Input: part model. Units: mm. Frame: model coordinates. A direction names the side the tool comes from. Give positions to 0.01 mm unless a question says otherwise; leave off trailing zeros. Loops run counter-clockwise (first coordinate to the right, second up) from the corner with the lowest first, then second, coordinate; pieces in that order, holes last. Notation, with made-up numbers: (10, -38.75) - (37, -38.75) arc R30 ccw to (37, -5.75) - close; hole circle Ø9 at (19.25, 66). An arc over 180 degrees is marked (long way). One line per item, written item: value.
from build123d import *

# Parameters (mm, degrees)
SKETCH_2_W               = 28
SKETCH_2_H               = 4.5
CUT_EXTRUDE_1_DEPTH      = 10
EXTRUDE_1_DEPTH          = 15
HOLE_WIZARD_M3_1_D       = 2.5
HOLE_WIZARD_M3_1_DEPTH   = 4
HOLE_WIZARD_M3_1_TIP     = 0.751075774
CUT_EXTRUDE_START        = -20
CUT_EXTRUDE_2_DEPTH      = 20
HOLE_WIZARD_M4_1_D       = 3.3
HOLE_WIZARD_M4_1_DEPTH   = 10.1
HOLE_WIZARD_M4_1_TIP     = 0.991420021
CUT_EXTRUDE_3_DEPTH      = 64.617293246
CUT_EXTRUDE_3_DEPTH_BACK = 64.617293246
SKETCH_11_R              = 1.5


with BuildPart() as part:
    # 草图1 → 旋转1 (revolve)
    with BuildSketch(Plane.XY, mode=Mode.PRIVATE) as revolve_1_sk:
        Polygon((0, 0), (4.1, 0), (4.1, 6.7), (13.4, 6.7), (13.4, 8.7), (21, 8.7), (21, 10.2), (20, 10.2), (20, 11.2), (21, 11.2), (21, 12.2), (10, 12.2), (10, 13.2), (21, 13.2), (21, 20.4), (5, 20.4), (5, 21), (21, 21), (21, 34.7), (18.3, 38.7), (3.5, 38.7), (3.5, 43.7), (0, 43.7), align=None)
    revolve(revolve_1_sk.sketch.rotate(Axis((0, 43.7, 0), (0, -1, 0)), 90), axis=Axis((0, 43.7, 0), (0, -1, 0)))

    # 草图2 → 切除-拉伸1 (cut)
    with BuildSketch(Plane.XY.offset(21)):
        with Locations((0, 16.05)):
            Rectangle(SKETCH_2_W, SKETCH_2_H)
    extrude(amount=-CUT_EXTRUDE_1_DEPTH, mode=Mode.SUBTRACT)

    # 草图3 → 凸台-拉伸1 (add)
    with BuildSketch(Plane.XY.offset(11)):
        with BuildLine():
            Line((9.185056323, 18.053194417), (9.385056323, 18.053194417))
            ThreePointArc((9.385056323, 18.053194417), (11.385056323, 16.053194417), (9.385056323, 14.053194417))
            Line((9.385056323, 14.053194417), (9.185056323, 14.053194417))
            ThreePointArc((9.185056323, 14.053194417), (7.185056323, 16.053194417), (9.185056323, 18.053194417))
        make_face()
    extrude(amount=EXTRUDE_1_DEPTH)

    # M3 螺纹孔1
    with Locations(Plane(origin=(0, 38.7, 0), x_dir=(1, 0, 0), z_dir=(0, 1, 0))):
        with Locations((-6.5, 0), (6.5, 0)):
            Hole(HOLE_WIZARD_M3_1_D / 2, depth=HOLE_WIZARD_M3_1_DEPTH)
            with Locations((0, 0, -(HOLE_WIZARD_M3_1_DEPTH + HOLE_WIZARD_M3_1_TIP / 2))):  # 118° drill point
                Cone(0, HOLE_WIZARD_M3_1_D / 2, HOLE_WIZARD_M3_1_TIP, mode=Mode.SUBTRACT)

    # 草图7 → 旋转2 (revolve)
    with BuildSketch(Plane.XY, mode=Mode.PRIVATE) as revolve_2_sk:
        Polygon((0, -54.6), (5, -54.6), (5, -30.5), (8.275, -30.5), (8.275, -29.6), (13, -29.6), (13, -27.6), (21, -27.6), (21, 8.7), (0, 8.7), align=None)
    revolve(revolve_2_sk.sketch.rotate(Axis((0, 8.7, 0), (0, -1, 0)), 180), axis=Axis((0, 8.7, 0), (0, -1, 0)))

    # 草图8 → 切除-拉伸2 (cut)
    with BuildSketch(Plane.XZ.offset(54.6).offset(CUT_EXTRUDE_START)):
        with BuildLine():
            Line((-3, 4), (3, 4))
            ThreePointArc((3, 4), (0, 5), (-3, 4))
        make_face()
    extrude(amount=CUT_EXTRUDE_2_DEPTH, mode=Mode.SUBTRACT)

    # M4 螺纹孔1
    with Locations(Plane(origin=(0, -27.6, 0), x_dir=(-1, 0, 0), z_dir=(0, -1, 0))):
        with Locations((0, -17.5), (-17.5, 0), (0, 17.5), (17.5, 0)):
            Hole(HOLE_WIZARD_M4_1_D / 2, depth=HOLE_WIZARD_M4_1_DEPTH)
            with Locations((0, 0, -(HOLE_WIZARD_M4_1_DEPTH + HOLE_WIZARD_M4_1_TIP / 2))):  # 118° drill point
                Cone(0, HOLE_WIZARD_M4_1_D / 2, HOLE_WIZARD_M4_1_TIP, mode=Mode.SUBTRACT)

    # 草图11 → 切除-拉伸3 (cut, two sides: drawn at the far end of the back side and taken through both)
    with BuildSketch(Plane.XY.offset(4).offset(-CUT_EXTRUDE_3_DEPTH_BACK)):
        with Locations((0, -44.6)):
            Circle(SKETCH_11_R)
    extrude(amount=CUT_EXTRUDE_3_DEPTH + CUT_EXTRUDE_3_DEPTH_BACK, mode=Mode.SUBTRACT)


solid = part.part
Item 1: Material intervals for L1, parallel to Y at x = 3.5, z = -14; L2, parallel to Z at x = 0, y = -24; L3, parallel to Y at x = 1, z = 16, sorted ascending.
Verdict:
L1: y = -27.6 to 12.2, 13.2 to 20.4, 21 to 38.7
L2: z = -21 to -19.15, -15.85 to 15.85, 19.15 to 21
L3: y = -27.6 to 12.2, 13.2 to 13.8, 18.3 to 20.4, 21 to 38.7
Item 2: Access query for faces 4 (the face through (0, 18.3, 15)), 5 (the face through (2, -44, 4)), 6 (the face through (-5.25, 36.67, -0.05)), 7 (the face through (4, -30.5, 4)), 8 (the face through (4, 20.4, 4)). Directions: +Z, -Z, +X, -X, +Y, -Y. A direction counts if a zero-diameter tool reaches every point of the face in a straight line with its end or side. Return the directions, or none.
Verdict:
face 4: +Z
face 5: +Z, +X, -X, -Y
face 6: +Y
face 7: -Y
face 8: none
Item 3: Section A-A, the plane y = -40. Output: boundary loops of the cut face in (x, z).
Verdict:
outline: (-3, 4) arc R5 ccw (long way) to (3, 4) - close
Item 4: Section D-D, the plane y = 16. Output: boundary loops of the cut face in (x, z), and give its area (3 significant figures).
Verdict:
outline: (-14, 11) - (-14, 15.65) arc R21 ccw (long way) to (14, 15.65) - (14, 11) - (11.38, 11) - (11.38, 26) - (7.19, 26) - (7.19, 11) - close
area: 1,220 mm^2
Item 5: Pin query (flat end, axial travel): P1, Ø3.5, axis at x = 0, y = -44.6, coming from the -Z side; P2, Ø1, axis at x = 10.5, y = 23, coming from the -Z side; P3, Ø3, axis at x = 14.5, y = 4, coming from the -Z side. Return the tip coordinate at first contact, or that it passes through.
Verdict:
P1: stops at z = -5
P2: stops at z = -18.47
P3: stops at z = -16.49
Item 6: Section B-B, the plane z = -11.5. Count the separate pieces of the cut face and the enclosed holes in it, and give its area (3 significant figures).
Verdict:
separate pieces: 3
enclosed holes: 0
area: 2,280 mm^2
Item 7: Draft query along X for faces 1 (the face through (4, 38.7, 0)), 2 (the face through (7.75, 36.67, -0.05)), 3 (the face through (-0.92, 16.85, -20.98)). Return one class per face: pulls with the +X half, pulls with the -X half, needs draft (parallel to the pull), parting line crosses it, or undercut.
Verdict:
face 1: needs draft
face 2: undercut
face 3: parting line crosses it
Item 8: Section C-C, the plane z = 22. Output: boundary loops of the cut face in (x, y).
Verdict:
outline: (9.19, 14.05) - (9.39, 14.05) arc R2 ccw to (9.39, 18.05) - (9.19, 18.05) arc R2 ccw to start
